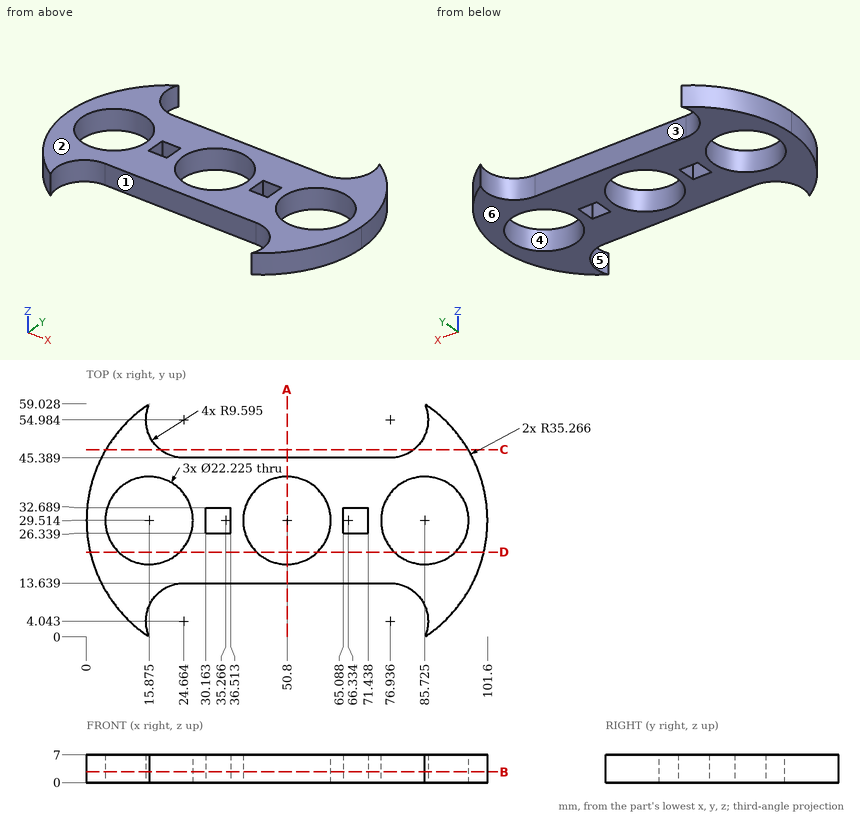
Answer from the drawing. Dimensions are ordinates in mm from the lowest x, y and z of the part. A direction names the side the tool comes from. Coordinates: 2 decimals unless noted, no trailing zeros. Write each loop counter-clockwise with the first axis right and the second up, starting at its lowest first coordinate (ties: lowest second). Pieces come first, ordered by that corner, then holes. Notation, with made-up numbers: (39, 82) - (82, 82) arc R9 ccw to (82, 94) - close; hole circle Ø4 at (2.5, -36.75). An arc over 180 degrees is marked (long way). One line per question, with ' | ' between items.
Q1. Find section B-B, the plane z = 2.75. Write down the section's boundary in (x, y) (1 decimal), plus the area to 3 significant figures.
Result set:
outline: (0, 29.5) arc R35.3 ccw to (16, 0) arc R9.6 cw to (24.7, 13.6) - (76.9, 13.6) arc R9.6 cw to (85.6, 0) arc R35.3 ccw to (101.6, 29.5) arc R35.3 ccw to (85.6, 59) arc R9.6 cw to (76.9, 45.4) - (24.7, 45.4) arc R9.6 cw to (16, 59) arc R35.3 ccw to start; hole circle Ø22.2 at (15.9, 29.5); hole (30.2, 26.3) - (36.5, 26.3) - (36.5, 32.7) - (30.2, 32.7) - close; hole circle Ø22.2 at (50.8, 29.5); hole (65.1, 26.3) - (71.4, 26.3) - (71.4, 32.7) - (65.1, 32.7) - close; hole circle Ø22.2 at (85.7, 29.5) | area: 2,330 mm^2
Q2. Determine the mould class of the marked faces 1, 2, 3 and 4 for opening direction Y: +Y half, -Y half, draft (parallel to the pull), parting line (faces both ways), or undercut.
Result set:
face 1: -Y half | face 2: draft | face 3: +Y half | face 4: undercut
Q3. Find section C-C, the plane y = 47.5. Write down the section's boundary in (x, z).
Result set:
outline: (4.93, 0) - (18.66, 0) - (18.66, 7) - (4.93, 7) - close; (82.94, 0) - (96.67, 0) - (96.67, 7) - (82.94, 7) - close
Q4. Find section A-A, the plane x = 50.8. Write down the section's boundary in (y, z).
Result set:
outline: (13.64, 0) - (18.4, 0) - (18.4, 7) - (13.64, 7) - close; (40.63, 0) - (45.39, 0) - (45.39, 7) - (40.63, 7) - close
Q5. Each of these flat-tipped pins is pushed along its axis until it touches: P1, Ø1.9, axis at x = 33.5, z = 3, coming from the -Y side; P2, Ø1.9, axis at x = 34.5, z = 2.5, coming from the +Y side; P3, Ø3, axis at x = 79.5, z = 1.5, coming from the +Y side. Where does it stop, or does it pass through?
Result set:
P1: y = 13.64 | P2: y = 45.39 | P3: y = 46.29
Q6. Consider L1, parallel to Y at x = 69, z = 6.25; L2, parallel to X at y = 25.5, z = 4.75; L3, parallel to X at y = 39, z = 3.5 (1 decimal). Determine where each line is inside the solid, lowest interval first. Write a range as [from, to].
Result set:
L1: [13.64, 26.34], [32.69, 45.39] | L2: [0.23, 5.51], [26.24, 40.44], [61.16, 75.36], [96.09, 101.37] | L3: [1.3, 10.1], [21.7, 45], [56.6, 79.9], [91.5, 100.3]
Q7. For the marked faces 5 and 6, determine the directions among +Z, -Z, +X, -X, +Y, -Y from which every point of the face is accessible in a straight line to the end or side of a thin tool.
Result set:
face 5: +Z, -Z | face 6: -Z, +X, -X, +Y, -Y
Q8. Find section D-D, the plane y = 21.5. Write down the section's boundary in (x, z), plus the area to 3 significant figures.
Result set:
outline: (0.92, 0) - (8.18, 0) - (8.18, 7) - (0.92, 7) - close; (23.57, 0) - (43.1, 0) - (43.1, 7) - (23.57, 7) - close; (58.5, 0) - (78.03, 0) - (78.03, 7) - (58.5, 7) - close; (93.42, 0) - (100.68, 0) - (100.68, 7) - (93.42, 7) - close | area: 375 mm^2
